from build123d import *

# Parameters (mm, degrees)
F1_DEPTH = 2
F2_R     = 5
F4_DEPTH = 208


with BuildPart() as f1:
    # F0 (on Front) → F1 (new body, symmetric)
    with BuildSketch(Plane.XZ):
        Polygon((-75, 30), (-75, 0), (-74, 0), (-73.5, 24.994999), (-71.5, 24.994999), (-71, 0), (-69, 0), (-68.5, 24.994999), (-66.5, 24.994999), (-66, 0), (-64, 0), (-63.5, 24.994999), (-61.5, 24.994999), (-61, 0), (-59, 0), (-58.5, 24.994999), (-56.5, 24.994999), (-56, 0), (-54, 0), (-53.5, 24.994999), (-51.5, 24.994999), (-51, 0), (-49, 0), (-48.5, 24.994999), (-46.5, 24.994999), (-46, 0), (-44, 0), (-43.5, 24.994999), (-41.5, 24.994999), (-41, 0), (-39, 0), (-38.5, 24.994999), (-36.5, 24.994999), (-36, 0), (-34, 0), (-33.5, 24.994999), (-31.5, 24.994999), (-31, 0), (-29, 0), (-28.5, 24.994999), (-26.5, 24.994999), (-26, 0), (-24, 0), (-23.5, 24.994999), (-21.5, 24.994999), (-21, 0), (-19, 0), (-18.5, 24.994999), (-16.5, 24.994999), (-16, 0), (-14, 0), (-13.5, 24.994999), (-11.5, 24.994999), (-11, 0), (-9, 0), (-8.5, 24.994999), (-6.5, 24.994999), (-6, 0), (-4, 0), (-3.5, 24.994999), (-1.5, 24.994999), (-1, 0), (0, 0), (0, 30), align=None)
    extrude(amount=F1_DEPTH, both=True)

    # F2
    f2_edges = [f1.edges().sort_by_distance(p)[0] for p in [
        (-75, 0, 30),
    ]]
    fillet(f2_edges, radius=F2_R)

    # F3 (on Right) → F4 (cut)
    with BuildSketch(Plane.YZ):
        Polygon((-1.037374, 0), (-2, 19.114297), (-2, 0), align=None)
    extrude(amount=-F4_DEPTH, mode=Mode.SUBTRACT)

    # F5: F1 across face


with BuildPart() as f1_1:
    add(f1.part)
    add(f1.part.mirror(Plane(origin=(0, 0.139421, 15.716448), x_dir=(0, 1, 0), z_dir=(1, 0, 0))))


solid = f1_1.part
Geometry check sheet. Reference: the model listing, model coordinates, mm. Round coordinates to 2 decimals unless told otherwise and drop trailing zeros. One line per question, with ' | ' between items. Start each with the question number.
(1) Thickness scan on L1, parallel to Z at x = 12, y = -0.7 (3 decimals); L2, parallel to X at y = -0.35, z = 25.5; L3, parallel to Y at x = -26, z = 18.75. Record the ranges inside material, lowest first. Write a range as [from, to].
(2) Depth check by flat-ended pin: pin 1 Ø4 at (x, z) = (-56, 5) entering from -Y; pin 2 Ø0.6 at (x, y) = (-47.5, -0.5) entering from -Z (3 decimals); pin 3 Ø4 at (x, z) = (20.5, 13) entering from -Y; pin 4 Ø5 at (x, z) = (-28.5, 22) entering from +Y. Enter the tip coordinate at first touch or a pass-through.
(3) Sectioned sample at A-A on z = 8.5. Count the separate pieces of the cut face and the enclosed holes in it, and give its area (3 significant figures).
Conclusion:
1) L1: z = [24.995, 30] | L2: x = [-74.97, 74.97] | L3: y = [-1.98, 2]
2) pin 1: stops at y = -1.39 | pin 2: stops at z = 24.995 | pin 3: stops at y = -1.79 | pin 4: stops at y = 2
3) separate pieces: 31 | enclosed holes: 0 | area: 243 mm2
